The model under review builds one solid part; all positions refer to its coordinate system, in mm. Coordinates: 2 decimals unless noted, no trailing zeros. Order: outer loops, then holes, each group sorted by start corner. A loop starts at its lowest first (then second) coordinate and runs counter-clockwise, first axis right, second up. Notation, with made-up numbers: (-31, 49) -> (-15, 49) arc R11 ccw to (-15, 65) -> close; hole circle Ø1 at (-14, 38.25). An arc over 180 degrees is marked (long way). Answer as CSV lines item,"result". Start each with the question number.
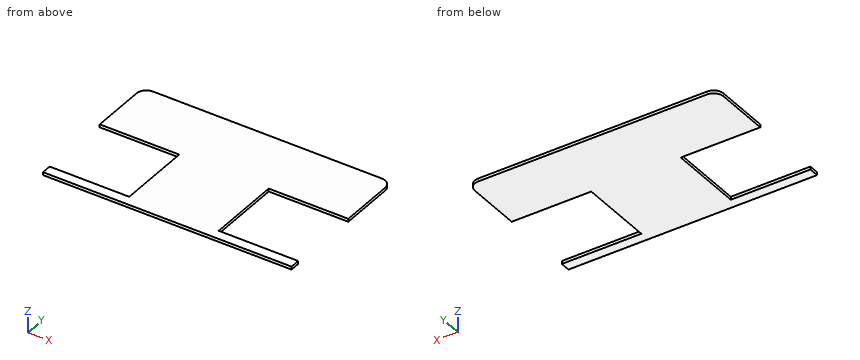
from build123d import *

# Parameters (mm, degrees)
BOSS_EXTRUDE1_DEPTH = 3


with BuildPart() as part:
    # Sketch1 → Boss-Extrude1 (new body)
    with BuildSketch(Plane.XY):
        with BuildLine():
            Line((10, 0), (240, 0))
            ThreePointArc((240, 0), (247.071067812, -2.928932188), (250, -10))
            Line((250, -10), (250, -65))
            Line((250, -65), (170, -65))
            Line((170, -65), (170, -140))
            Line((170, -140), (250, -140))
            Line((250, -140), (250, -150))
            Line((250, -150), (0, -150))
            Line((0, -150), (0, -140))
            Line((0, -140), (80, -140))
            Line((80, -140), (80, -65))
            Line((80, -65), (0, -65))
            Line((0, -65), (0, -10))
            ThreePointArc((0, -10), (2.928932188, -2.928932188), (10, 0))
        make_face()
    extrude(amount=BOSS_EXTRUDE1_DEPTH)


solid = part.part
1) Consider section C-C (y = -112.5). Give the boundary of the cut face in (x, z), plus the area to 3 significant figures.
2) Wall thickness on L1, parallel to Y at x = 63.5, z = 2.6; L2, parallel to X at y = -105.5, z = 1.1; L3, parallel to X at y = -9.5, z = 0.2: over which ranges is each line inside the solid? List them lowest first. Write a range as [from, to].
3) Consider section A-A (x = 225.5). Give the boundary of the cut face in (y, z), plus the area to 3 significant figures.
4) Insertion check: pin 1 Ø4 at (x, y) = (158.5, -117) entering from -Z. The pin has a flat end and moves straight along its axis. Give the tip position at first contact, or say it passes through.
5) Consider section B-B (z = 0.7). Give the boundary of the cut face in (x, y).
Result:
1,outline,"(80, 0) -> (170, 0) -> (170, 3) -> (80, 3) -> close"
1,area,"270 mm2"
2,L1,"[-150, -140], [-65, 0]"
2,L2,"[80, 170]"
2,L3,"[0.01, 249.99]"
3,outline,"(-150, 0) -> (-140, 0) -> (-140, 3) -> (-150, 3) -> close; (-65, 0) -> (0, 0) -> (0, 3) -> (-65, 3) -> close"
3,area,"225 mm2"
4,pin 1,"z = 0"
5,outline,"(0, -150) -> (250, -150) -> (250, -140) -> (170, -140) -> (170, -65) -> (250, -65) -> (250, -10) arc R10 ccw to (240, 0) -> (10, 0) arc R10 ccw to (0, -10) -> (0, -65) -> (80, -65) -> (80, -140) -> (0, -140) -> close"
